For this review, take the finished solid that the model builds, in its own axes (mm). A direction names the side the tool comes from. Round coordinates to 2 decimals unless told otherwise and drop trailing zeros. Order: outer loops, then holes, each group sorted by start corner. A loop starts at its lowest first (then second) coordinate and runs counter-clockwise, first axis right, second up. Notation, with made-up numbers: (17.5, 57) -> (48.5, 57) arc R18 ccw to (48.5, 88) -> close; hole circle Ø10 at (0, 76). An arc over 180 degrees is marked (long way). Answer in a Markdown table with one row per item.
Autodesk Inventor part; units mm, degrees
ref_plane "YZ Plane" through (0, 0, 0) normal (1, 0, 0) x (0, 1, 0)
ref_plane "XZ Plane" through (0, 0, 0) normal (0, 1, 0) x (-1, 0, 0)
ref_plane "XY Plane" through (0, 0, 0) normal (0, 0, 1) x (1, 0, 0)
sketch "Sketch1" plane through (0, 0, 0) normal (0, 1, 0) x (-1, 0, 0)
  line L0 (-18.2565, -12.5) -> (18.2565, -12.5)
  line L1 (18.2565, -12.5) -> (18.2565, 12.5)
  line L2 (18.2565, 12.5) -> (-18.2565, 12.5)
  line L3 (-18.2565, 12.5) -> (-18.2565, -12.5)
  line L4 (-18.2565, -12.5) -> (18.2565, 12.5) construction
  line L5 (18.2565, -12.5) -> (-18.2565, 12.5) construction
  point P0 (0, 0)
  dimension "d0" = 36.513
  dimension "d1" = 25
extrude "Extrusion1" add sketch "Sketch1" against normal blind 5
sketch "Sketch2" plane through (18.2565, 0, 12.5) normal (1, 0, 0) x (0, 0, -1)
  circle A0 centre (30, 0) radius 5
  line L0 (25, 0) -> (25, -5)
  line L1 (25, -5) -> (0, -5)
  line L2 (0, -5) -> (25, -5)
  line L3 (25, -5) -> (30, -5)
  line L4 (30, -5) -> (30, 0)
  line L5 (30, 0) -> (25, 0)
  line L6 (25, 0) -> (25, -5)
  point P0 (12.5, 0)
  dimension "d4" = 5
  dimension "d5" = 10
  dimension "d6" = 5
extrude "Extrusion2" add sketch "Sketch2" against normal blind 36.513
sketch "Sketch3" plane through (18.2565, -5, 12.5) normal (1, 0, 0) x (0, 0, -1)
  circle A0 centre (30, 5) radius 2.5
  line L0 (0, 0) -> (30, 0)
  line L1 (0, 5) -> (0, 0)
  point P0 (12.5, 5)
  dimension "d9" = 5
  dimension "d10" = 30
  dimension "d11" = 5
extrude "Extrusion3" cut sketch "Sketch3" against normal blind 36.513
sketch "Sketch4" plane through (0, -5, 0) normal (0, -1, 0) x (1, 0, 0)
  line L0 (18.2565, 12.5) -> (18.2565, -17.5)
  line L1 (18.2565, -9.5) -> (8.2565, -9.5)
  line L2 (8.2565, -9.5) -> (8.2565, -22.5)
  line L3 (8.2565, -22.5) -> (18.2565, -22.5)
  line L4 (18.2565, -22.5) -> (18.2565, -9.5)
  line L5 (-18.2565, -9.5) -> (-8.2565, -9.5)
  line L6 (-8.2565, -9.5) -> (-8.2565, -22.5)
  line L7 (-8.2565, -22.5) -> (-18.2565, -22.5)
  line L8 (-18.2565, -22.5) -> (-18.2565, -9.5)
  line L9 (18.2565, -17.5) -> (-18.2565, -17.5)
  line L10 (-18.2565, 12.5) -> (-18.2565, -17.5)
  point P0 (0, 0)
  point P1 (18.2565, -17.5)
  dimension "d14" = 5
  dimension "d15" = 16.513
  dimension "d16" = 0
  dimension "d17" = 10
  dimension "d18" = 13
extrude "Extrusion4" cut sketch "Sketch4" against normal blind 36.513
properties part number "hinge 2" material "Stainless Steel"
Q1. To check wall thickness, follow probe 1 along Y at (x, z) = (1.5, -17.5); probe 2 along X at (y, z) = (3, -18); probe 3 along Z at (x, y) = (14.5, -0.5). State the ranges of each line that lie inside material, in increasing order.
Answer key:
| item | result |
|---|---|
| probe 1 | y = -5 to -2.5, 2.5 to 5 |
| probe 2 | x = -8.26 to 8.26 |
| probe 3 | z = -9.5 to 12.5 |
Q2. Take a section at A-A, the plane x = -1. Write out the cut boundary in (y, z).
Answer key:
| item | result |
|---|---|
| outline | (-5, -17.5) arc R5 ccw (long way) to (0, -12.5) -> (0, 12.5) -> (-5, 12.5) -> close; hole circle Ø5 at (0, -17.5) |
Q3. Take a section at D-D, the plane y = -3. Write out the cut boundary in (x, z), then the cut area to 3 significant figures.
Answer key:
| item | result |
|---|---|
| outline | (-18.26, -9.5) -> (-8.26, -9.5) -> (-8.26, -21.5) -> (8.26, -21.5) -> (8.26, -9.5) -> (18.26, -9.5) -> (18.26, 12.5) -> (-18.26, 12.5) -> close |
| area | 1,000 mm^2 |
Q4. Take a section at C-C, the plane z = -16.5. Write out the cut boundary in (x, y), then the cut area to 3 significant figures.
Answer key:
| item | result |
|---|---|
| outline | (-8.26, -5) -> (8.26, -5) -> (8.26, -2.29) -> (-8.26, -2.29) -> close; (-8.26, 2.29) -> (8.26, 2.29) -> (8.26, 4.9) -> (-8.26, 4.9) -> close |
| area | 87.8 mm^2 |
Q5. Clearance check with flat-ended pins moving along their axes: pin 1 Ø3 at (x, y) = (10, -1.5) entering from -Z; pin 2 Ø5 at (x, y) = (4.5, 1.5) entering from +Z; pin 3 Ø3 at (y, z) = (2.5, -15) entering from -X; pin 4 Ø1.5 at (y, z) = (2, -18.5) entering from +X. State where each tip first meets the part, or that it passes through.
Answer key:
| item | result |
|---|---|
| pin 1 | stops at z = -9.5 |
| pin 2 | stops at z = 12.5 |
| pin 3 | stops at x = -8.26 |
| pin 4 | stops at x = 8.26 |
Q6. The part is to be moulded in two halves that separate along Y. For faces 1 (the face through (0, 0, -15)), 2 (the face through (0, 0, 0)), 3 (the face through (0.12, 3.42, -21.15)), 4 (the face through (0, -2, 12.5)), say which applies: +Y half, -Y half, draft (parallel to the pull), parting line (faces both ways), or undercut.
Answer key:
| item | result |
|---|---|
| face 1 | undercut |
| face 2 | +Y half |
| face 3 | parting line |
| face 4 | draft |
Q7. Take a section at B-B, the plane y = 1.25. Write out the cut boundary in (x, z), then the cut area to 3 significant figures.
Answer key:
| item | result |
|---|---|
| outline | (-8.26, -22.34) -> (8.26, -22.34) -> (8.26, -19.67) -> (-8.26, -19.67) -> close; (-8.26, -15.33) -> (8.26, -15.33) -> (8.26, -12.66) -> (-8.26, -12.66) -> close |
| area | 88.4 mm^2 |
Q8. Tool access review of faces 5 (the face through (-13, -3, -9.5)), 6 (the face through (0, -5, -2)), 7 (the face through (8.256, -1, -14)): name each direction out of +Z, -Z, +X, -X, +Y, -Y from which nothing blocks a thin tool from reaching the whole face with its end or side.
Answer key:
| item | result |
|---|---|
| face 5 | -Z, -X, +Y, -Y |
| face 6 | +Z, -Z, +X, -X, -Y |
| face 7 | -Z, +X, +Y, -Y |
